from build123d import *

# Parameters (mm, degrees)
CROQUIS2_W                   = 160
CROQUIS2_H                   = 160
CROQUIS2_W_2                 = 140
CROQUIS2_H_2                 = 140
SALIENTE_EXTRUIR1_DEPTH      = 10
CROQUIS3_W                   = 152
CROQUIS3_H                   = 152
CROQUIS3_W_2                 = 150
CROQUIS3_H_2                 = 150
CROQUIS3_W_3                 = 148
CROQUIS3_H_3                 = 148
CORTAR_EXTRUIR1_DEPTH        = 3.5
CROQUIS4_W                   = 10
CROQUIS4_H                   = 10
SALIENTE_EXTRUIR2_DEPTH      = 140
SALIENTE_EXTRUIR2_DEPTH_BACK = 10
CROQUIS7_W                   = 160
CROQUIS7_H                   = 160
CROQUIS7_W_2                 = 140
CROQUIS7_H_2                 = 140
SALIENTE_EXTRUIR3_DEPTH      = 10
CROQUIS8_W                   = 63
CROQUIS8_H                   = 12
CROQUIS8_R                   = 2.5
SALIENTE_EXTRUIR4_DEPTH      = 5
CROQUIS9_W                   = 10
CROQUIS9_H                   = 160
CORTAR_EXTRUIR2_DEPTH        = 161


with BuildPart() as part:
    # Croquis2 → Saliente-Extruir1 (new body)
    with BuildSketch(Plane.XY):
        with Locations((80, -80)):
            Rectangle(CROQUIS2_W, CROQUIS2_H)
        with Locations((80, -80)):
            Rectangle(CROQUIS2_W_2, CROQUIS2_H_2, mode=Mode.SUBTRACT)
    extrude(amount=SALIENTE_EXTRUIR1_DEPTH)

    # Croquis3 → Cortar-Extruir1 (cut)
    with BuildSketch(Plane.XY.offset(10)):
        with Locations((80, -80)):
            Rectangle(CROQUIS3_W, CROQUIS3_H)
        with Locations((80, -80)):
            Rectangle(CROQUIS3_W_2, CROQUIS3_H_2, mode=Mode.SUBTRACT)
        with Locations((80, -80)):
            Rectangle(CROQUIS3_W_2, CROQUIS3_H_2)
        with Locations((80, -80)):
            Rectangle(CROQUIS3_W_3, CROQUIS3_H_3, mode=Mode.SUBTRACT)
    extrude(amount=-CORTAR_EXTRUIR1_DEPTH, mode=Mode.SUBTRACT)

    # Croquis4 → Saliente-Extruir2 (add, two sides)
    with BuildSketch(Plane.XY.offset(10)) as saliente_extruir2_sk:
        with Locations((5, -5)):
            Rectangle(CROQUIS4_W, CROQUIS4_H)
        with Locations((155, -5)):
            Rectangle(CROQUIS4_W, CROQUIS4_H)
        with Locations((155, -155)):
            Rectangle(CROQUIS4_W, CROQUIS4_H)
        with Locations((5, -155)):
            Rectangle(CROQUIS4_W, CROQUIS4_H)
    extrude(amount=SALIENTE_EXTRUIR2_DEPTH)
    extrude(saliente_extruir2_sk.sketch, amount=-SALIENTE_EXTRUIR2_DEPTH_BACK)

    # Croquis7 → Saliente-Extruir3 (add)
    with BuildSketch(Plane.XY.offset(150)):
        with Locations((80, -80)):
            Rectangle(CROQUIS7_W, CROQUIS7_H)
        with Locations((80, -80)):
            Rectangle(CROQUIS7_W_2, CROQUIS7_H_2, mode=Mode.SUBTRACT)
    extrude(amount=SALIENTE_EXTRUIR3_DEPTH)

    # Croquis8 → Saliente-Extruir4 (add)
    with BuildSketch(Plane.XY.offset(160)):
        with Locations((31.5, -80)):
            Rectangle(CROQUIS8_W, CROQUIS8_H)
        with Locations((55, -80)):
            Circle(CROQUIS8_R, mode=Mode.SUBTRACT)
        with Locations((128.5, -80)):
            Rectangle(CROQUIS8_W, CROQUIS8_H)
        with Locations((105, -80)):
            Circle(CROQUIS8_R, mode=Mode.SUBTRACT)
    extrude(amount=-SALIENTE_EXTRUIR4_DEPTH)

    # Croquis9 → Cortar-Extruir2 (cut, through all)
    with BuildSketch(Plane.ZY):
        with Locations((5, -80)):
            Rectangle(CROQUIS9_W, CROQUIS9_H)
    extrude(amount=-CORTAR_EXTRUIR2_DEPTH, mode=Mode.SUBTRACT)


solid = part.part
The model under review builds one solid part; all positions refer to its coordinate system, in mm. A direction names the side the tool comes from. Coordinates: 2 decimals unless noted, no trailing zeros. Loops run counter-clockwise (first coordinate to the right, second up) from the corner with the lowest first, then second, coordinate; pieces in that order, holes last. Notation, with made-up numbers: (26, 30.5) -> (45, 30.5) arc R32 cw to (45, 64.5) -> close; hole circle Ø7 at (60.5, 49.25). An arc over 180 degrees is marked (long way). Use a Markdown table: item, result. Add a question column.
1. Clearance check with flat-ended pins moving along their axes: pin 1 Ø13 at (x, y) = (48, -78) entering from -Z; pin 2 Ø5 at (x, y) = (95.5, -6) entering from -Z. State where each tip first meets the part, or that it passes through.
2. Machinability: for faces 3 (the face through (79, -155, 150)), 4 (the face through (155, -150, 79)), 5 (the face through (123, -80, 155)), which of the approach directions +Z, -Z, +X, -X, +Y, -Y give a long, thin tool a straight path to every point of the face, cutting with its end or side? Answer none if there is none.
3. Add section A-A on z = 29.5. Write out the cut boundary in (x, y).
4. Add section D-D on y = -28. Write out the cut boundary in (x, z), plus the area to 3 significant figures.
5. To check wall thickness, follow line 1 (Y direction, x = 55, z = 158.5); line 2 (Y direction, x = 151.5, z = 51.5); line 3 (Z direction, x = 146, y = -8). State the ranges of each line that lie inside material, in increasing order.
6. Draft analysis for pull direction Y (two halves, no side actions). For faces 1 (the face through (36, -80, 155)), 2 (the face through (150, -155, 79)), state which applies: pulls with the +Y half, pulls with the -Y half, needs draft (parallel to the pull), parting line crosses it, or undercut.
7. Add section C-C on y = -80. Write out the cut boundary in (x, z).
8. Add section B-B on x = 55. Write out the cut boundary in (y, z), plus the area to 3 significant figures.
Returned:
| question | item | result |
|---|---|---|
| 1 | pin 1 | stops at z = 155 |
| 1 | pin 2 | stops at z = 150 |
| 2 | face 3 | -Z, +Y, -Y |
| 2 | face 4 | -Z, +X, -X |
| 2 | face 5 | -Z |
| 3 | outline | (0, -160) -> (10, -160) -> (10, -150) -> (0, -150) -> close; (0, -10) -> (10, -10) -> (10, 0) -> (0, 0) -> close; (150, -160) -> (160, -160) -> (160, -150) -> (150, -150) -> close; (150, -10) -> (160, -10) -> (160, 0) -> (150, 0) -> close |
| 4 | outline | (0, 150) -> (10, 150) -> (10, 160) -> (0, 160) -> close; (150, 150) -> (160, 150) -> (160, 160) -> (150, 160) -> close |
| 4 | area | 200 mm² |
| 5 | line 1 | y = -160 to -150, -86 to -82.5, -77.5 to -74, -10 to 0 |
| 5 | line 2 | y = -160 to -150, -10 to 0 |
| 5 | line 3 | z = 150 to 160 |
| 6 | face 1 | undercut |
| 6 | face 2 | needs draft |
| 7 | outline | (0, 150) -> (10, 150) -> (10, 155) -> (52.5, 155) -> (52.5, 160) -> (0, 160) -> close; (57.5, 155) -> (63, 155) -> (63, 160) -> (57.5, 160) -> close; (97, 155) -> (102.5, 155) -> (102.5, 160) -> (97, 160) -> close; (107.5, 155) -> (150, 155) -> (150, 150) -> (160, 150) -> (160, 160) -> (107.5, 160) -> close |
| 8 | outline | (-160, 150) -> (-150, 150) -> (-150, 160) -> (-160, 160) -> close; (-86, 155) -> (-82.5, 155) -> (-82.5, 160) -> (-86, 160) -> close; (-77.5, 155) -> (-74, 155) -> (-74, 160) -> (-77.5, 160) -> close; (-10, 150) -> (0, 150) -> (0, 160) -> (-10, 160) -> close |
| 8 | area | 235 mm² |
